Autodesk Inventor part; units mm, degrees
ref_plane "YZ Plane" through (0, 0, 0) normal (1, 0, 0) x (0, 1, 0)
ref_plane "XZ Plane" through (0, 0, 0) normal (0, 1, 0) x (-1, 0, 0)
ref_plane "XY Plane" through (0, 0, 0) normal (0, 0, 1) x (1, 0, 0)
sketch "Sketch1" plane through (0, 0, 0) normal (0, 1, 0) x (-1, 0, 0)
  line L0 (-7.62, 190.5) -> (7.62, 190.5)
  line L1 (7.62, 190.5) -> (7.62, -190.5)
  line L2 (7.62, -190.5) -> (-7.62, -190.5)
  line L3 (-7.62, -190.5) -> (-7.62, 190.5)
  line L4 (-7.62, 190.5) -> (7.62, -190.5) construction
  line L5 (7.62, 190.5) -> (-7.62, -190.5) construction
  point P0 (0, 0)
  dimension "d0" = 15.24
  dimension "d1" = 381
extrude "Extrusion1" add sketch "Sketch1" along normal blind 12.7
sketch "Sketch2" plane through (0, 12.7, 0) normal (0, 1, 0) x (1, 0, 0)
  line L0 (-7.62, 190.5) -> (-7.62, -190.5)
  line L1 (-7.62, -139.7) -> (-20.32, -139.7)
  line L2 (-20.32, -139.7) -> (-20.32, -127)
  line L3 (-20.32, -127) -> (-7.62, -127)
  line L4 (-7.62, -127) -> (-7.62, -139.7)
  circle A0 centre (-13.97, -133.35) radius 3.175
  point P0 (0, 0)
  dimension "d4" = 12.7
  dimension "d5" = 12.7
  dimension "d6" = 127
  dimension "d7" = 6.35
  dimension "d8" = 6.35
  dimension "d9" = 6.35
extrude "Extrusion2" add sketch "Sketch2" against normal up to surface (12.7 mm away)
mirror "Mirror1" about plane through (0, 0, 0) normal (1, 0, 0) of "Extrusion2"
mirror "Mirror2" about plane through (0, 0, 0) normal (0, 0, 1) of "Extrusion2", "Mirror1"
equation "\"d8\" = 0.5 * d4"
equation "\"d9\" = 0.5 * d5"
properties part number "Rack Bottom"
Source: CAD feature listing. Evaluate the final solid. Frame: model axes, mm. A direction names the side the tool comes from. Round coordinates to 2 decimals unless told otherwise and drop trailing zeros. Order: outer loops, then holes, each group sorted by start corner. A loop starts at its lowest first (then second) coordinate and runs counter-clockwise, first axis right, second up. Notation, with made-up numbers: (-27, -5.75) - (-2, -5.75) arc R8 ccw to (-2, 0.25) - close; hole circle Ø9 at (9.5, 51). An arc over 180 degrees is marked (long way). Use a Markdown table: item, result. Add a question column.
1. Section query B-B (z = -133.35). Return the cut outline in (x, y) (3 decimals), then the cut area to 3 significant figures.
2. Section query A-A (x = -13.97). Return the cut outline in (y, z) (3 decimals), then the cut area to 3 significant figures.
3. Set-up query: faces 1 (the flat face through (14, 6, 127)), 2 (the flat face through (-14, 6, 127)), 3 (the flat face through (14, 6, -139.7)), 4 (the flat face through (-14, 6, 139.7)). Return all of +Z, -Z, +X, -X, +Y, -Y with unobstructed straight access to the full face (end or side cutting, diameter ignored); none if empty.
4. Mould query, pull axis X, two halves, no side actions, for faces 5 (the cylindrical face through (14.66, 6.44, -136.45)), 6 (the flat face through (20.32, 6, -133)), 7 (the flat face through (0, 12.7, 45)), 8 (the cylindrical face through (14.66, 6.44, 130.25)). Classes: +X half, -X half, draft (parallel to the pull), parting line (faces both ways), or undercut.
5. First-contact query: pin 1 (3 mm diameter, centred on y = 7.5, z = 36, fed in from -X); pin 2 (6.5 mm diameter, centred on y = 7, z = -14.5, fed in from +X); pin 3 (4 mm diameter, centred on x = -16, y = 6, fed in from +Z). Flat tips, straight axial feed; report the tip coordinate or a pass-through.
6. Section query C-C (y = 4.5). Return the cut outline in (x, z) (3 decimals).
7. Section query D-D (z = -21). Return the cut outline in (x, y).
8. Line query: probe 1 along X at (y, z) = (10, -133.35) (3 decimals); probe 2 along Z at (x, y) = (-13.97, 5.5) (3 decimals); probe 3 along Z at (x, y) = (-15.5, 11.75). Output: solid intervals per line, ascending.
Derived:
| question | item | result |
|---|---|---|
| 1 | outline | (-20.32, 0) - (-17.145, 0) - (-17.145, 12.7) - (-20.32, 12.7) - close; (-10.795, 0) - (10.795, 0) - (10.795, 12.7) - (-10.795, 12.7) - close; (17.145, 0) - (20.32, 0) - (20.32, 12.7) - (17.145, 12.7) - close |
| 1 | area | 355 mm2 |
| 2 | outline | (0, -139.7) - (12.7, -139.7) - (12.7, -136.525) - (0, -136.525) - close; (0, -130.175) - (12.7, -130.175) - (12.7, -127) - (0, -127) - close; (0, 127) - (12.7, 127) - (12.7, 130.175) - (0, 130.175) - close; (0, 136.525) - (12.7, 136.525) - (12.7, 139.7) - (0, 139.7) - close |
| 2 | area | 161 mm2 |
| 3 | face 1 | +X, +Y, -Y |
| 3 | face 2 | -X, +Y, -Y |
| 3 | face 3 | -Z, +X, +Y, -Y |
| 3 | face 4 | +Z, -X, +Y, -Y |
| 4 | face 5 | undercut |
| 4 | face 6 | +X half |
| 4 | face 7 | draft |
| 4 | face 8 | undercut |
| 5 | pin 1 | x = -7.62 |
| 5 | pin 2 | x = 7.62 |
| 5 | pin 3 | z = 139.7 |
| 6 | outline | (-20.32, -139.7) - (-7.62, -139.7) - (-7.62, -190.5) - (7.62, -190.5) - (7.62, -139.7) - (20.32, -139.7) - (20.32, -127) - (7.62, -127) - (7.62, 127) - (20.32, 127) - (20.32, 139.7) - (7.62, 139.7) - (7.62, 190.5) - (-7.62, 190.5) - (-7.62, 139.7) - (-20.32, 139.7) - (-20.32, 127) - (-7.62, 127) - (-7.62, -127) - (-20.32, -127) - close; hole circle Ø6.35 at (-13.97, -133.35); hole circle Ø6.35 at (-13.97, 133.35); hole circle Ø6.35 at (13.97, -133.35); hole circle Ø6.35 at (13.97, 133.35) |
| 7 | outline | (-7.62, 0) - (7.62, 0) - (7.62, 12.7) - (-7.62, 12.7) - close |
| 8 | probe 1 | -20.32 to -17.145, -10.795 to 10.795, 17.145 to 20.32 |
| 8 | probe 2 | -139.7 to -136.525, -130.175 to -127, 127 to 130.175, 136.525 to 139.7 |
| 8 | probe 3 | -139.7 to -136.13, -130.57 to -127, 127 to 130.57, 136.13 to 139.7 |
